Build history of the part. All positions in model axes, mm. A direction names the side the tool comes from. Round coordinates to 2 decimals unless told otherwise and drop trailing zeros. Loops run counter-clockwise (first coordinate to the right, second up) from the corner with the lowest first, then second, coordinate; pieces in that order, holes last. Notation, with made-up numbers: (-24, 50) - (1, 50) arc R16 cw to (1, 54) - close; hole circle Ø4 at (37, 46). An arc over 180 degrees is marked (long way). Use a Markdown table: item, result.
from build123d import *

# Parameters (mm, degrees)
BOSS_EXTRUDE1_DEPTH = 3.175


with BuildPart() as part:
    # Sketch1 → Boss-Extrude1 (new body)
    with BuildSketch(Plane.XY):
        Polygon((-1.6256, 18.923), (-1.6256, 63.5), (-4.1656, 63.5), (-25.4, 2.54), (-25.4, 0), (-19.05, 0), (-19.05, -3.81), (-6.35, -3.81), (-6.35, 0), (0, 0), (6.35, 0), (6.35, -3.81), (19.05, -3.81), (19.05, 0), (25.4, 0), (25.4, 2.54), (4.1656, 63.5), (1.6256, 63.5), (1.6256, 18.923), align=None)
    extrude(amount=BOSS_EXTRUDE1_DEPTH)


solid = part.part
Q1. Cut at D-D, the plane y = 5.5. List the corners of the cut face in (x, z) (3 decimals), plus the area to 3 significant figures.
Results found:
| item | result |
|---|---|
| outline | (-24.369, 0) - (24.369, 0) - (24.369, 3.175) - (-24.369, 3.175) - close |
| area | 155 mm2 |
Q2. Probe line 1 (Y direction, x = -3.5, z = 2.45); line 2 (Y direction, x = 1, z = 2.1); line 3 (X direction, y = 53, z = 2.4). List the from-to ranges inside material, lowest first.
Results found:
| item | result |
|---|---|
| line 1 | y = 0 to 63.5 |
| line 2 | y = 0 to 18.92 |
| line 3 | x = -7.82 to -1.63, 1.63 to 7.82 |
Q3. Cut at A-A, the plane y = 28. List the corners of the cut face in (x, z) (3 decimals), plus the area to 3 significant figures.
Results found:
| item | result |
|---|---|
| outline | (-16.531, 0) - (-1.626, 0) - (-1.626, 3.175) - (-16.531, 3.175) - close; (1.626, 0) - (16.531, 0) - (16.531, 3.175) - (1.626, 3.175) - close |
| area | 94.7 mm2 |
Q4. Cut at B-B, the plane z = 1. List the corners of the cut face in (x, y).
Results found:
| item | result |
|---|---|
| outline | (-25.4, 0) - (-19.05, 0) - (-19.05, -3.81) - (-6.35, -3.81) - (-6.35, 0) - (6.35, 0) - (6.35, -3.81) - (19.05, -3.81) - (19.05, 0) - (25.4, 0) - (25.4, 2.54) - (4.17, 63.5) - (1.63, 63.5) - (1.63, 18.92) - (-1.63, 18.92) - (-1.63, 63.5) - (-4.17, 63.5) - (-25.4, 2.54) - close |
Q5. Pull direction X, two halves, no side cores. Call faces 5 (the face through (19.05, -2, 2)), 6 (the face through (-25.4, 1, 2)), 7 (the face through (0, 15, 3.175)), 8 (the face through (-6.35, -2, 2)): pulls with the +X half, pulls with the -X half, needs draft (parallel to the pull), parting line crosses it, or undercut.
Results found:
| item | result |
|---|---|
| face 5 | pulls with the +X half |
| face 6 | pulls with the -X half |
| face 7 | needs draft |
| face 8 | undercut |
Q6. Drop flat-ended pins along their axis: pin 1 (1.6 mm diameter, centred on y = 40, z = 1.5, fed in from +X); pin 2 (1 mm diameter, centred on y = -1, z = 2, fed in from +X); pin 3 (1.6 mm diameter, centred on x = 22, z = 2, fed in from -Y). Give the stop position or say it passes through.
Results found:
| item | result |
|---|---|
| pin 1 | stops at x = 12.63 |
| pin 2 | stops at x = 19.05 |
| pin 3 | stops at y = 0 |
Q7. Cut at C-C, the plane x = -14. List the corners of the cut face in (y, z) (3 decimals), plus the area to 3 significant figures.
Results found:
| item | result |
|---|---|
| outline | (-3.81, 0) - (35.267, 0) - (35.267, 3.175) - (-3.81, 3.175) - close |
| area | 124 mm2 |
Q8. Which spindle directions (+Z, -Z, +X, -X, +Y, -Y) get a long thin tool onto all of the face, cutting with end or side? Do faces 1 (the face through (22, 0, 2)), 2 (the face through (1.626, 42, 2)), 3 (the face through (-22, 0, 2)), 4 (the face through (0, 0, 2)). Say none if no direction does.
Results found:
| item | result |
|---|---|
| face 1 | +Z, -Z, +X, -Y |
| face 2 | +Z, -Z, +Y |
| face 3 | +Z, -Z, -X, -Y |
| face 4 | +Z, -Z, -Y |
